For this review, take the finished solid that the model builds, in its own axes (mm). Face numbers are marked on the shaded views. A direction names the side the tool comes from. Coordinates: 2 decimals unless noted, no trailing zeros. Loops run counter-clockwise (first coordinate to the right, second up) from the corner with the lowest first, then second, coordinate; pieces in that order, holes last. Notation, with made-up numbers: (44.5, 30.5) -> (66.5, 30.5) arc R22 cw to (66.5, 61.5) -> close; hole circle Ø1 at (67.5, 88). An arc over 180 degrees is marked (long way). One line per item, written item: value.
from build123d import *

# Parameters (mm, degrees)
SKETCH_1_W                       = 40
SKETCH_1_H                       = 20
SM_BASE_FLANGE_1_DEPTH           = 2
SM_EDGE_FLANGE_1_STRIP_W         = 9.4732
SM_EDGE_FLANGE_1_STRIP_H         = 2
SM_EDGE_FLANGE_1_STRIP_CUT_DEPTH = 20
SM_EDGE_FLANGE_1_DEPTH           = 20
HOLE_WIZARD_M3_2_D               = 2.5
HOLE_WIZARD_3_5_3_5_2_D          = 3.5


# Sheet-metal steps are written as plain solids
with BuildPart() as part:
    # Sketch 1 → 基材-凸緣1 (new body)
    with BuildSketch(Plane.XY):
        Rectangle(SKETCH_1_W, SKETCH_1_H)
    extrude(amount=-SM_BASE_FLANGE_1_DEPTH)

    # 邊線-凸緣1 strip (across the edge) → 邊線-凸緣1 strip cut (cut)
    with BuildSketch(Plane(origin=(20, -10, 0), x_dir=(-1, 0, 0), z_dir=(0, 1, 0))):
        with Locations((-4, -1)):
            Rectangle(SM_EDGE_FLANGE_1_STRIP_W, SM_EDGE_FLANGE_1_STRIP_H)
    extrude(amount=SM_EDGE_FLANGE_1_STRIP_CUT_DEPTH, mode=Mode.SUBTRACT)

    # 邊線-凸緣1 section (across the edge) → 邊線-凸緣1 (add)
    with BuildSketch(Plane(origin=(20, -10, 0), x_dir=(-1, 0, 0), z_dir=(0, 1, 0))):
        with BuildLine():
            Line((-2, 0.7366), (-2, 10))
            Line((-2, 10), (0, 10))
            Line((0, 10), (0, 0.7366))
            ThreePointArc((0, 0.7366), (0.215745145, 0.215745145), (0.7366, 0))
            Line((0.7366, 0), (0.7366, -2))
            ThreePointArc((0.7366, -2), (-1.198468417, -1.198468417), (-2, 0.7366))
        make_face()
    extrude(amount=SM_EDGE_FLANGE_1_DEPTH)

    # M3 螺紋孔2 (through all)
    with Locations(Plane.XY):
        with Locations((-13.5, -5), (13.5, -5), (13.5, 5), (-13.5, 5)):
            Hole(HOLE_WIZARD_M3_2_D / 2)

    # Ø3.5 (3.5) 直徑孔2 (through all)
    with Locations(Plane(origin=(22, 0, 0), x_dir=(0, 0, -1), z_dir=(1, 0, 0))):
        with Locations((-6, 0)):
            Hole(HOLE_WIZARD_3_5_3_5_2_D / 2)


solid = part.part
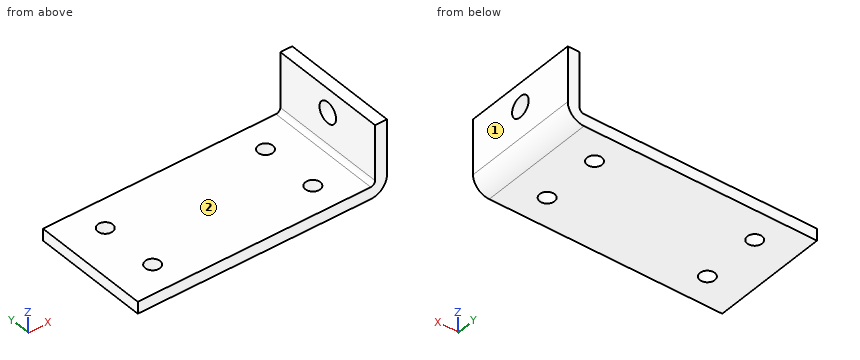
1. For the marked faces 1 and 2, list the 3-axis set-ups (+Z, -Z, +X, -X, +Y, -Y) from which the entire face can be reached by the end or side of a thin tool; tool diameter is ignored.
Return value:
face 1: +Z, -Z, +X, +Y, -Y
face 2: +Z, -X, +Y, -Y
2. To check wall thickness, follow probe 1 along Y at (x, z) = (-13.5, -1.4); probe 2 along Y at (x, z) = (20.7, 6); probe 3 along X at (y, z) = (-7.25, 8). State the ranges of each line that lie inside material, in increasing order. Write a range as from..to.
Return value:
probe 1: y = -10..-6.25, -3.75..3.75, 6.25..10
probe 2: y = -10..-1.75, 1.75..10
probe 3: x = 20..22
3. Insertion check: pin 1 Ø3 at (y, z) = (-1, 6) entering from +X; pin 2 Ø1.5 at (x, y) = (-13.5, 5) entering from +Z; pin 3 Ø1.5 at (y, z) = (3, 8.5) entering from -X; pin 4 Ø10 at (x, y) = (8.5, 0) entering from +Z. Each pin has a flat end and moves straight along its axis. Give the tip position at first contact, or say it passes through.
Return value:
pin 1: stops at x = 22
pin 2: passes through
pin 3: stops at x = 20
pin 4: stops at z = 0
4. Take a section at C-C, the plane z = 6. Give the boundary of the cut face in (x, y), and give its area (3 significant figures).
Return value:
outline: (20, -10) -> (22, -10) -> (22, -1.75) -> (20, -1.75) -> close; (20, 1.75) -> (22, 1.75) -> (22, 10) -> (20, 10) -> close
area: 33.0 mm2
5. Take a section at B-B, the plane y = -5. Give the boundary of the cut face in (x, z), and give its area (3 significant figures).
Return value:
outline: (-20, -2) -> (-14.75, -2) -> (-14.75, 0) -> (-20, 0) -> close; (-12.25, -2) -> (12.25, -2) -> (12.25, 0) -> (-12.25, 0) -> close; (14.75, -2) -> (19.26, -2) arc R2.74 ccw to (22, 0.74) -> (22, 10) -> (20, 10) -> (20, 0.74) arc R0.74 cw to (19.26, 0) -> (14.75, 0) -> close
area: 92.5 mm2
6. Take a section at D-D, the plane x = 13.5. Give the boundary of the cut face in (y, z), and give its area (3 significant figures).
Return value:
outline: (-10, -2) -> (-6.25, -2) -> (-6.25, 0) -> (-10, 0) -> close; (-3.75, -2) -> (3.75, -2) -> (3.75, 0) -> (-3.75, 0) -> close; (6.25, -2) -> (10, -2) -> (10, 0) -> (6.25, 0) -> close
area: 30.0 mm2
7. Take a section at A-A, the plane y = 0. Give the boundary of the cut face in (x, z), and give its area (3 significant figures).
Return value:
outline: (-20, -2) -> (19.26, -2) arc R2.74 ccw to (22, 0.74) -> (22, 4.25) -> (20, 4.25) -> (20, 0.74) arc R0.74 cw to (19.26, 0) -> (-20, 0) -> close; (20, 7.75) -> (22, 7.75) -> (22, 10) -> (20, 10) -> close
area: 95.5 mm2
